Can you work these out from the model? Positions are in its coordinate system, mm. A direction names the side the tool comes from. Give positions to 0.01 mm unless a question says otherwise; leave off trailing zeros. Loops run counter-clockwise (first coordinate to the right, second up) from the corner with the lowest first, then second, coordinate; pieces in that order, holes last.
from build123d import *

# Parameters (mm, degrees)
SKETCH_1_W          = 100
SKETCH_1_H          = 65
EXTRUDE_1_DEPTH     = 12
SKETCH_2_R          = 3.5
CUT_EXTRUDE_2_DEPTH = 10
SKETCH_3_R          = 3.5
CUT_EXTRUDE_3_DEPTH = 61.466933112
SKETCH_4_R          = 3.5
CUT_EXTRUDE_4_DEPTH = 61.466933112
CUT_EXTRUDE_5_REACH = 84.879
SKETCH_5_R          = 1.5
CUT_EXTRUDE_6_REACH = 84.879
SKETCH_6_R          = 1.5
FILLET_3_R          = 2
FILLET_4_R          = 4


with BuildPart() as part:
    # 草图1 → 凸台-拉伸1 (new body)
    with BuildSketch(Plane(origin=(0, 0, 0), x_dir=(1, 0, 0), z_dir=(0, 1, 0))):
        Rectangle(SKETCH_1_W, SKETCH_1_H)
    extrude(amount=EXTRUDE_1_DEPTH)

    # 草图2 → 切除-拉伸2 (cut)
    with BuildSketch(Plane(origin=(0, 12, 0), x_dir=(1, 0, 0), z_dir=(0, 1, 0))):
        with Locations(Location((-40, -9, 0), (0, 0, 270))):
            Circle(SKETCH_2_R)
        with Locations(Location((40, -9, 0), (0, 0, 90))):
            Circle(SKETCH_2_R)
        with BuildLine():
            Line((-30.422291236, 30.788854382), (-33.577708764, 29.211145618))
            ThreePointArc((-33.577708764, 29.211145618), (-34.012630114, 29.053502021), (-34.472135955, 29))
            Line((-34.472135955, 29), (-41, 29))
            ThreePointArc((-41, 29), (-43.828427125, 27.828427125), (-45, 25))
            Line((-45, 25), (-45, 6))
            ThreePointArc((-45, 6), (-43.535533906, 2.464466094), (-40, 1))
            ThreePointArc((-40, 1), (-30, -9), (-40, -19))
            ThreePointArc((-40, -19), (-45, -24), (-40, -29))
            Line((-40, -29), (-34.439229319, -29))
            ThreePointArc((-34.439229319, -29), (-33.976113717, -29.054357705), (-33.538172016, -29.214476061))
            Line((-33.538172016, -29.214476061), (-30.425003094, -30.785523939))
            ThreePointArc((-30.425003094, -30.785523939), (-29.987061393, -30.945642295), (-29.52394579, -31))
            Line((-29.52394579, -31), (29.52394579, -31))
            ThreePointArc((29.52394579, -31), (29.987061393, -30.945642295), (30.425003094, -30.785523939))
            Line((30.425003094, -30.785523939), (33.538172016, -29.214476061))
            ThreePointArc((33.538172016, -29.214476061), (33.976113717, -29.054357705), (34.439229319, -29))
            Line((34.439229319, -29), (40, -29))
            ThreePointArc((40, -29), (45, -24), (40, -19))
            ThreePointArc((40, -19), (30, -9), (40, 1))
            ThreePointArc((40, 1), (43.535533906, 2.464466094), (45, 6))
            Line((45, 6), (45, 25))
            ThreePointArc((45, 25), (43.828427125, 27.828427125), (41, 29))
            Line((41, 29), (34.472135955, 29))
            ThreePointArc((34.472135955, 29), (34.012630114, 29.053502021), (33.577708764, 29.211145618))
            Line((33.577708764, 29.211145618), (30.422291236, 30.788854382))
            ThreePointArc((30.422291236, 30.788854382), (29.987369886, 30.946497979), (29.527864045, 31))
            Line((29.527864045, 31), (-29.527864045, 31))
            ThreePointArc((-29.527864045, 31), (-29.987369886, 30.946497979), (-30.422291236, 30.788854382))
        make_face()
    extrude(amount=-CUT_EXTRUDE_2_DEPTH, mode=Mode.SUBTRACT)

    # 草图3 → 切除-拉伸3 (cut, through all)
    with BuildSketch(Plane(origin=(0, 2, 0), x_dir=(1, 0, 0), z_dir=(0, 1, 0))):
        with Locations(Location((-40, -9, 0), (0, 0, 270))):
            Circle(SKETCH_3_R)
    extrude(amount=-CUT_EXTRUDE_3_DEPTH, mode=Mode.SUBTRACT)

    # 草图4 → 切除-拉伸4 (cut, through all)
    with BuildSketch(Plane(origin=(0, 2, 0), x_dir=(1, 0, 0), z_dir=(0, 1, 0))):
        with Locations(Location((40, -9, 0), (0, 0, 270))):
            Circle(SKETCH_4_R)
    extrude(amount=-CUT_EXTRUDE_4_DEPTH, mode=Mode.SUBTRACT)

    # 草图5 → 切除-拉伸5 (cut, up to next)
    with BuildSketch(Plane.XY.offset(32.5), mode=Mode.PRIVATE) as cut_extrude_5_sk1:
        with Locations((-40, 6)):
            Circle(SKETCH_5_R)
    cut_extrude_5_tool1 = extrude(cut_extrude_5_sk1.sketch, amount=-CUT_EXTRUDE_5_REACH, mode=Mode.PRIVATE) & part.part
    # 草图5 → 切除-拉伸5 (cut, up to next)
    with BuildSketch(Plane.XY.offset(32.5), mode=Mode.PRIVATE) as cut_extrude_5_sk2:
        with Locations((40, 6)):
            Circle(SKETCH_5_R)
    cut_extrude_5_tool2 = extrude(cut_extrude_5_sk2.sketch, amount=-CUT_EXTRUDE_5_REACH, mode=Mode.PRIVATE) & part.part
    add(cut_extrude_5_tool1.solids().sort_by_distance((-40, 6, 32.5))[0], mode=Mode.SUBTRACT)
    add(cut_extrude_5_tool2.solids().sort_by_distance((40, 6, 32.5))[0], mode=Mode.SUBTRACT)

    # 草图6 → 切除-拉伸6 (cut, up to next)
    with BuildSketch(Plane(origin=(0, 0, -32.5), x_dir=(-1, 0, 0), z_dir=(0, 0, -1)), mode=Mode.PRIVATE) as cut_extrude_6_sk1:
        with Locations(Location((-40, 6, 0), (0, 0, 180))):
            Circle(SKETCH_6_R)
    cut_extrude_6_tool1 = extrude(cut_extrude_6_sk1.sketch, amount=-CUT_EXTRUDE_6_REACH, mode=Mode.PRIVATE) & part.part
    # 草图6 → 切除-拉伸6 (cut, up to next)
    with BuildSketch(Plane(origin=(0, 0, -32.5), x_dir=(-1, 0, 0), z_dir=(0, 0, -1)), mode=Mode.PRIVATE) as cut_extrude_6_sk2:
        with Locations(Location((40, 6, 0), (0, 0, 180))):
            Circle(SKETCH_6_R)
    cut_extrude_6_tool2 = extrude(cut_extrude_6_sk2.sketch, amount=-CUT_EXTRUDE_6_REACH, mode=Mode.PRIVATE) & part.part
    add(cut_extrude_6_tool1.solids().sort_by_distance((40, 6, -32.5))[0], mode=Mode.SUBTRACT)
    add(cut_extrude_6_tool2.solids().sort_by_distance((-40, 6, -32.5))[0], mode=Mode.SUBTRACT)

    # 圆角3
    fillet_3_edges = [part.edges().sort_by_distance(p)[0] for p in [
        (-50, 12, 0),
        (50, 12, 0),
    ]]
    fillet(fillet_3_edges, radius=FILLET_3_R)

    # 圆角4
    fillet_4_edges = [part.edges().sort_by_distance(p)[0] for p in [
        (-50, 0, 0),
        (50, 0, 0),
    ]]
    fillet(fillet_4_edges, radius=FILLET_4_R)


solid = part.part
(1) Thinking about a two-plate mould opening in X: for faces 4 (the flat face through (-50, 7, 0)), 5 (the flat face through (0, 7, 31)), 6 (the flat face through (-1, 6, -32.5)), which applies, pulls with the +X half, pulls with the -X half, needs draft (parallel to the pull), parting line crosses it, or undercut?
Returned:
face 4: pulls with the -X half
face 5: undercut
face 6: needs draft
(2) Suppose I cut it at D-D on x = -2.5. List the corners of the cut face in (y, z) for me, plus the area to 3 significant figures.
Returned:
outline: (0, -32.5) - (12, -32.5) - (12, -31) - (2, -31) - (2, 31) - (12, 31) - (12, 32.5) - (0, 32.5) - close
area: 160 mm2
(3) Suppose I cut it at C-C on y = 6. Give the number of separate pieces and of enclosed holes in the cut face, plus the area to 3 significant figures.
Returned:
separate pieces: 4
enclosed holes: 2
area: 1,460 mm2
(4) Suppose I cut it at B-B on z = 24. List the corners of the cut face in (x, y) for me, plus the area to 3 significant figures.
Returned:
outline: (-50, 4) arc R4 ccw to (-46, 0) - (46, 0) arc R4 ccw to (50, 4) - (50, 10) arc R2 ccw to (48, 12) - (45, 12) - (45, 2) - (-45, 2) - (-45, 12) - (-48, 12) arc R2 ccw to (-50, 10) - close
area: 291 mm2
(5) Please list where these lines run through material, in increasing order: probe 1 along X at (y, z) = (6, 31.45); probe 2 along Z at (x, y) = (-1, 7.5); probe 3 along Y at (x, z) = (40, 29.7).
Returned:
probe 1: x = -50 to -41.5, -38.5 to 38.5, 41.5 to 50
probe 2: z = -32.5 to -31, 31 to 32.5
probe 3: y = 0 to 4.5, 7.5 to 12
(6) Suppose I cut it at A-A on z = 9. List the corners of the cut face in (x, y) for me, plus the area to 3 significant figures.
Returned:
outline: (-50, 4) arc R4 ccw to (-46, 0) - (-43.5, 0) - (-43.5, 12) - (-48, 12) arc R2 ccw to (-50, 10) - close; (-36.5, 0) - (36.5, 0) - (36.5, 12) - (30, 12) - (30, 2) - (-30, 2) - (-30, 12) - (-36.5, 12) - close; (43.5, 0) - (46, 0) arc R4 ccw to (50, 4) - (50, 10) arc R2 ccw to (48, 12) - (43.5, 12) - close
area: 423 mm2
(7) Will these pins go through, and if not, where does the flat tip stop? P1, Ø12, axis at x = -19, z = -5, coming from the +Y side; P2, Ø1.8, axis at x = -40, y = 6, coming from the +Z side.
Returned:
P1: stops at y = 2
P2: stops at z = 19.08
(8) Which directions (+Z, -Z, +X, -X, +Y, -Y) give clear straight access to the entire face, cutting with the end or side of a thin tool? Please do faces 1 (the flat face through (50, 7, 0)), 2 (the flat face through (-45, 7, -16)), 3 (the cylindrical face through (-41.5, 6.07, 30.66)).
Returned:
face 1: +Z, -Z, +X, +Y, -Y
face 2: +Y
face 3: +Z
